Input: part model. Units: mm. Frame: model coordinates. A direction names the side the tool comes from. Round coordinates to 2 decimals unless told otherwise and drop trailing zeros. Loops run counter-clockwise (first coordinate to the right, second up) from the corner with the lowest first, then second, coordinate; pieces in that order, holes last. Notation, with made-up numbers: (32, 53.5) - (86, 53.5) arc R12 ccw to (86, 69.5) - close; hole circle Ø2 at (39.25, -33.5). An arc over 180 degrees is marked (long way). One line per question, with ' | ' between items. Start each with the question number.
from build123d import *

# Parameters (mm, degrees)
SKETCH_2_W           = 20
SKETCH_2_H           = 14
EXTRUDE_1_DEPTH      = 18
SKETCH_6_R           = 4.4
CUT_EXTRUDE_4_DEPTH  = 1.5
DOME_1_FACE_RADIUS   = 4.4
DOME_1_HEIGHT        = 1
SKETCH_7_W           = 0.5
SKETCH_7_H           = 18
CUT_EXTRUDE_5_DEPTH  = 20
SKETCH_8_W           = 4
SKETCH_8_H           = 18
CUT_EXTRUDE_6_DEPTH  = 27
SKETCH_12_W          = 18
SKETCH_12_H          = 11
CUT_EXTRUDE_9_DEPTH  = 4
SKETCH_13_R          = 2
SKETCH_13_R_2        = 1.15
CUT_EXTRUDE_10_DEPTH = 15.5
SKETCH_14_R          = 4.4
CUT_EXTRUDE_11_DEPTH = 1
CHAMFER_1_SIZE       = 1
FILLET_1_R           = 1


with BuildPart() as part:
    # 草图2 → 凸台-拉伸1 (new body)
    with BuildSketch(Plane.XY):
        Rectangle(SKETCH_2_W, SKETCH_2_H)
    extrude(amount=EXTRUDE_1_DEPTH)

    # 草图6 → 切除-拉伸4 (cut)
    with BuildSketch(Plane.XZ.offset(7)):
        with Locations(Location((0, 9, 0), (0, 0, 270))):
            Circle(SKETCH_6_R)
    extrude(amount=-CUT_EXTRUDE_4_DEPTH, mode=Mode.SUBTRACT)

    # 圆顶1: a dome of height H over a round flat face of radius A is a cap of a sphere of radius (A * A + H * H) / (2 * H)
    dome_1_r = (DOME_1_FACE_RADIUS * DOME_1_FACE_RADIUS + DOME_1_HEIGHT * DOME_1_HEIGHT) / (2 * DOME_1_HEIGHT)
    dome_1_base = Plane((0, -5.5, 9), z_dir=(0, 1, 0))
    with Locations(dome_1_base.offset(DOME_1_HEIGHT - dome_1_r)):
        dome_1_ball = Sphere(dome_1_r, mode=Mode.PRIVATE)
    add(split(dome_1_ball, bisect_by=dome_1_base, keep=Keep.TOP, mode=Mode.PRIVATE), mode=Mode.SUBTRACT)

    # 草图7 → 切除-拉伸5 (cut)
    with BuildSketch(Plane.XZ.offset(7)):
        with Locations((9.75, 9)):
            Rectangle(SKETCH_7_W, SKETCH_7_H)
    extrude(amount=-CUT_EXTRUDE_5_DEPTH, mode=Mode.SUBTRACT)

    # 草图8 → 切除-拉伸6 (cut)
    with BuildSketch(Plane.XZ.offset(7)):
        with Locations((-8, 9)):
            Rectangle(SKETCH_8_W, SKETCH_8_H)
    extrude(amount=-CUT_EXTRUDE_6_DEPTH, mode=Mode.SUBTRACT)

    # 草图12 → 切除-拉伸9 (cut)
    with BuildSketch(Plane.ZY.offset(6)):
        with Locations((9, 1.5)):
            Rectangle(SKETCH_12_W, SKETCH_12_H)
    extrude(amount=-CUT_EXTRUDE_9_DEPTH, mode=Mode.SUBTRACT)

    # 草图13 → 切除-拉伸10 (cut)
    with BuildSketch(Plane.ZY.offset(2)):
        with Locations((9, 1.5)):
            Circle(SKETCH_13_R)
        with Locations((3, 1.5)):
            Circle(SKETCH_13_R_2)
        with Locations((15, 1.5)):
            Circle(SKETCH_13_R_2)
    extrude(amount=-CUT_EXTRUDE_10_DEPTH, mode=Mode.SUBTRACT)

    # 草图14 → 切除-拉伸11 (cut)
    with BuildSketch(Plane.ZY.offset(2)):
        with Locations((9, 1.5)):
            Circle(SKETCH_14_R)
    extrude(amount=-CUT_EXTRUDE_11_DEPTH, mode=Mode.SUBTRACT)

    # 倒角1
    chamfer_1_edges = [part.edges().sort_by_distance(p)[0] for p in [
        (9.5, 1.5, 13.85),
        (9.5, 1.5, 1.85),
    ]]
    chamfer(chamfer_1_edges, length=CHAMFER_1_SIZE)

    # 圆角1
    fillet_1_edges = [part.edges().sort_by_distance(p)[0] for p in [
        (3.75, 7, 0),
        (3.75, 7, 18),
        (1.75, -7, 0),
        (1.75, -7, 18),
        (-6, -5.5, 0),
        (-6, -5.5, 18),
    ]]
    fillet(fillet_1_edges, radius=FILLET_1_R)


solid = part.part
(1) Reachability of faces 1 (the face through (4, 0, 18)), 2 (the face through (1.322, -6.26, 4.803)), 3 (the face through (-4, -4, 9)), 4 (the face through (-1.507, 2.822, 13.197)) from +Z, -Z, +X, -X, +Y, -Y: full face, straight path, thin tool, end or side. Return the list, or none.
(2) Section B-B, the plane z = 15. Output: boundary loops of the cut face in (x, y), plus the area to 3 significant figures.
(3) Line query: line 1 along Y through (x, z) = (0.75, 3); line 2 along Z through (x, y) = (4.25, 0.5); line 3 along Z through (x, y) = (7.25, 1). Output: solid intervals per line, ascending. Write a range as from..to.
(4) Section C-C, the plane x = 0. Output: boundary loops of the cut face in (y, z).
(5) Pull-direction query (Y, two-part tool) for faces 5 (the face through (-1, 4, 9)), 6 (the face through (1.859, -6.715, 17.699)), 7 (the face through (3.83, 6.699, 17.715)), 8 (the face through (-2, -1, 13)); classes: released by +Y, released by -Y, zero draft, split by the parting line, or undercut.
(6) Section A-A, the plane y = 1.5. Output: boundary loops of the cut face in (x, z), plus the area to 3 significant figures.
(7) Pin query (flat end, axial travel): P1, Ø4.5, axis at y = 1.5, z = 8.5, coming from the -X side; P2, Ø1.2, axis at x = -4, z = 6, coming from the +Y side; P3, Ø2, axis at y = 1.5, z = 3, coming from the -X side; P4, Ø2.5, axis at y = 1.5, z = 15, coming from the +X side. Return the tip coordinate at first contact, or that it passes through.
(8) Section D-D, the plane z = 9. Output: boundary loops of the cut face in (x, y), plus the area to 3 significant figures.
Derived:
1) face 1: +Z, +X, -X, +Y, -Y | face 2: -Y | face 3: +Z, -Z, -X, +Y | face 4: -X
2) outline: (-6, -7) - (9.5, -7) - (9.5, -0.65) - (8.5, 0.35) - (-2, 0.35) - (-2, -4) - (-6, -4) - close; (-2, 2.65) - (8.5, 2.65) - (9.5, 3.65) - (9.5, 7) - (-2, 7) - close | area: 146 mm²
3) line 1: y = -7..0.35, 2.65..7 | line 2: z = 0..2.43, 3.57..7.27, 10.73..14.43, 15.57..18 | line 3: z = 0..1.96, 4.04..7.06, 10.94..13.96, 16.04..18
4) outline: (-7, 1) arc R1 ccw to (-6, 0) - (6, 0) arc R1 ccw to (7, 1) - (7, 17) arc R1 ccw to (6, 18) - (-6, 18) arc R1 ccw to (-7, 17) - (-7, 13.4) - (-5.5, 13.4) arc R10.18 cw to (-5.5, 4.6) - (-7, 4.6) - close; hole circle Ø4 at (1.5, 9); hole circle Ø2.3 at (1.5, 3); hole circle Ø2.3 at (1.5, 15)
5) face 5: undercut | face 6: released by -Y | face 7: released by +Y | face 8: zero draft
6) outline: (-2, 0) - (9.5, 0) - (9.5, 0.85) - (8.5, 1.85) - (-2, 1.85) - close; (-2, 4.15) - (8.5, 4.15) - (9.5, 5.15) - (9.5, 7) - (-1, 7) - (-1, 4.6) - (-2, 4.6) - close; (-2, 13.4) - (-1, 13.4) - (-1, 11) - (9.5, 11) - (9.5, 12.85) - (8.5, 13.85) - (-2, 13.85) - close; (-2, 16.15) - (8.5, 16.15) - (9.5, 17.15) - (9.5, 18) - (-2, 18) - close | area: 101 mm²
7) P1: stops at x = -1 | P2: stops at y = -4 | P3: passes through | P4: stops at x = 8.6
8) outline: (-6, -7) - (-4.4, -7) - (-4.4, -5.5) arc R10.18 cw to (4.4, -5.5) - (4.4, -7) - (9.5, -7) - (9.5, -0.5) - (-1, -0.5) - (-1, -2.9) - (-2, -2.9) - (-2, -4) - (-6, -4) - close; (-2, 5.9) - (-1, 5.9) - (-1, 3.5) - (9.5, 3.5) - (9.5, 7) - (-2, 7) - close | area: 103 mm²
